Work out the finished part from the listing and answer in its coordinate system (mm). Give positions to 0.01 mm unless a question says otherwise; leave off trailing zeros. Order: outer loops, then holes, each group sorted by start corner. A loop starts at its lowest first (then second) coordinate and runs counter-clockwise, first axis right, second up. Notation, with made-up numbers: (32, 57) -> (66, 57) arc R26 cw to (66, 77) -> close; hole circle Ø11 at (51.5, 41). An arc over 180 degrees is marked (long way). Answer as CSV lines item,"result". Start each with the question number.
1. A cutting plane is placed at C-C (y = 2). State how many separate pieces and enclosed holes the cut face has, then the cut area to 3 significant figures.
2. A cutting plane is placed at D-D (z = -38). Give the vertices of the cut face in (x, y), then the cut area to 3 significant figures.
3. A cutting plane is placed at A-A (z = 27.5). Give the vertices of the cut face in (x, y).
4. A cutting plane is placed at B-B (x = -16). Give the vertices of the cut face in (y, z) (3 decimals), then the cut area to 3 significant figures.
5. Find the intervals of material crossed by L1, parallel to Z at x = -16, y = 1.9 (3 decimals); L2, parallel to Z at x = 4.5, y = 2.25; L3, parallel to Z at x = -32.5, y = 2.65, in increasing order.
6. Flat-ended cylindrical pins translate along their axes: pin 1 (2.5 mm diameter, centred on x = 30, z = 54, fed in from +Y); pin 2 (2.5 mm diameter, centred on x = -32, z = 55, fed in from +Y); pin 3 (0.9 mm diameter, centred on y = 2, z = 0.5, fed in from +X); pin 4 (1.5 mm diameter, centred on y = 1, z = -17, fed in from -X). Find the tip coordinate at first contact, or state that the pin passes through.
Autodesk Inventor part; units mm, degrees
ref_plane "YZ Plane" through (0, 0, 0) normal (1, 0, 0) x (0, 1, 0)
ref_plane "XZ Plane" through (0, 0, 0) normal (0, 1, 0) x (-1, 0, 0)
ref_plane "XY Plane" through (0, 0, 0) normal (0, 0, 1) x (1, 0, 0)
sketch "Sketch1" plane through (0, 0, 0) normal (0, 1, 0) x (-1, 0, 0)
  line L0 (32, 55) -> (-32, 55)
  line L1 (-32, 55) -> (-32, -55)
  line L2 (-32, -55) -> (32, -55)
  line L3 (32, -55) -> (32, 55)
  line L4 (32, 55) -> (-32, -55) construction
  line L5 (-32, 55) -> (32, -55) construction
  circle A0 centre (32, 55) radius 4.2425
  circle A1 centre (32, -55) radius 4.2425
  circle A2 centre (-32, 55) radius 4.2425
  circle A3 centre (-32, -55) radius 4.2425
  point P0 (0, 0)
  dimension "d0" = 64
  dimension "d1" = 110
  dimension "d2" = 8.485
  dimension "d5" = 110
  dimension "d8" = 64
extrude "Extrusion1" add sketch "Sketch1" along normal blind 3
sketch "Sketch2" plane through (0, 3, 0) normal (0, 1, 0) x (1, 0, 0)
  line L0 (32, -50.7575) -> (32, 50.7575)
  arc A0 (32, 50.7575) -> (27.7575, 55) centre (32, 55) ccw
  line L1 (27.7575, 55) -> (-27.7575, 55)
  arc A1 (-27.7575, 55) -> (-32, 50.7575) centre (-32, 55) ccw
  line L2 (-32, 50.7575) -> (-32, -50.7575)
  arc A2 (-32, -50.7575) -> (-27.7575, -55) centre (-32, -55) ccw
  line L3 (-27.7575, -55) -> (27.7575, -55)
  arc A3 (27.7575, -55) -> (32, -50.7575) centre (32, -55) ccw
  circle A4 centre (-32, -55) radius 2.15
  circle A5 centre (-32, 55) radius 2.15
  circle A6 centre (32, -55) radius 2.15
  circle A7 centre (32, 55) radius 2.15
  point P0 (0, 0)
  dimension "d13" = 4.3
  dimension "d16" = 110
  dimension "d19" = 64
extrude "Extrusion2" cut sketch "Sketch2" against normal blind 3 contours A4 | A5 | A6 | A7
sketch "Sketch3" plane through (0, 3, 0) normal (0, 1, 0) x (1, 0, 0)
  line L0 (-8, -38.5) -> (8, -38.5)
  line L1 (8, -38.5) -> (8, -5.5)
  line L2 (8, -5.5) -> (-8, -5.5)
  line L3 (-8, -5.5) -> (-8, -38.5)
  line L4 (-32, 50.7575) -> (-32, -50.7575)
  line L5 (32, -50.7575) -> (32, 50.7575)
  line L6 (-27.7575, -55) -> (27.7575, -55)
  point P0 (0, 0)
  dimension "d24" = 16
  dimension "d25" = 33
  dimension "d26" = 24
  dimension "d27" = 24
  dimension "d28" = 16.5
extrude "Extrusion3" cut sketch "Sketch3" against normal blind 3
sketch "Sketch4" plane through (0, 3, 0) normal (0, 1, 0) x (1, 0, 0)
  circle A0 centre (-16, 9.625) radius 3.4
  line L0 (0, 82.9395) -> (0, -82.9395)
  circle A1 centre (-16, 24.75) radius 3.4
  circle A2 centre (-16, 39.875) radius 3.4
  line L1 (27.7575, 55) -> (-27.7575, 55)
  line L2 (-8, -5.5) -> (8, -5.5)
  line L3 (-16, 0) -> (-16, 55)
  circle A3 centre (9, 25) radius 6
  line L4 (32, -50.7575) -> (32, 50.7575)
  point P0 (0, 0)
  dimension "d31" = 6.8
  dimension "d32" = 6.8
  dimension "d33" = 6.8
  dimension "d34" = 15.125
  dimension "d35" = 15.125
  dimension "d36" = 15.125
  dimension "d37" = 15.125
  dimension "d53" = 16
  dimension "d54" = 55
  dimension "d55" = 12
  dimension "d56" = 23
  dimension "d64" = 30
extrude "Extrusion4" cut sketch "Sketch4" against normal blind 6
sketch "Sketch5" plane through (0, 3, 0) normal (0, 1, 0) x (1, 0, 0)
  circle A0 centre (-16, 24.75) radius 3.4
  circle A1 centre (-16, 9.625) radius 3.4
  circle A2 centre (-16, 39.875) radius 3.4
  line L0 (8, -5.5) -> (8, -38.5)
  line L1 (8, -38.5) -> (-8, -38.5)
  line L2 (-8, -38.5) -> (-8, -5.5)
  line L3 (-8, -5.5) -> (8, -5.5)
  circle A3 centre (32, -55) radius 2.15
  circle A4 centre (-32, -55) radius 2.15
  circle A5 centre (-32, 55) radius 2.15
  circle A6 centre (32, 55) radius 2.15
  line L4 (32, -50.7575) -> (32, 50.7575)
  arc A7 (32, 50.7575) -> (27.7575, 55) centre (32, 55) ccw
  line L5 (27.7575, 55) -> (-27.7575, 55)
  arc A8 (-27.7575, 55) -> (-32, 50.7575) centre (-32, 55) ccw
  line L6 (-32, 50.7575) -> (-32, -50.7575)
  arc A9 (-32, -50.7575) -> (-27.7575, -55) centre (-32, -55) ccw
  line L7 (-27.7575, -55) -> (27.7575, -55)
  arc A10 (27.7575, -55) -> (32, -50.7575) centre (32, -55) ccw
  circle A11 centre (-32, -55) radius 2.15
  circle A12 centre (-32, -55) radius 4.2425
  circle A13 centre (-32, 55) radius 4.2425
  circle A14 centre (32, -55) radius 4.2425
  circle A15 centre (32, 55) radius 4.2425
  line L8 (-32, -50.7575) -> (-32, 50.7575)
  line L9 (-27.7575, 55) -> (27.7575, 55)
  line L10 (32, -50.7575) -> (32, 50.7575)
  line L11 (32, 50.7575) -> (32, -50.7575)
  line L12 (-27.7575, -55) -> (27.7575, -55)
  line L13 (27.7575, -55) -> (-27.7575, -55)
  circle A16 centre (-16, 39.875) radius 3.4
  circle A17 centre (-16, 9.625) radius 3.4
  circle A18 centre (-16, 24.75) radius 3.4
  circle A19 centre (9, 25) radius 6
  line L14 (8, -38.5) -> (8, -5.5)
  line L15 (8, -5.5) -> (-8, -5.5)
  line L16 (-8, -5.5) -> (-8, -38.5)
  line L17 (-8, -38.5) -> (8, -38.5)
  circle A20 centre (32, -55) radius 2.15
  circle A21 centre (-32, -55) radius 2.15
  circle A22 centre (-32, 55) radius 2.15
  circle A23 centre (32, 55) radius 2.15
  line L18 (-27.7575, -55) -> (27.7575, -55)
  arc A24 (-32, -50.7575) -> (-27.7575, -55) centre (-32, -55) ccw
  line L19 (-32, 50.7575) -> (-32, -50.7575)
  arc A25 (-27.7575, 55) -> (-32, 50.7575) centre (-32, 55) ccw
  line L20 (27.7575, 55) -> (-27.7575, 55)
  arc A26 (32, 50.7575) -> (27.7575, 55) centre (32, 55) ccw
  line L21 (32, -50.7575) -> (32, 50.7575)
  arc A27 (27.7575, -55) -> (32, -50.7575) centre (32, -55) ccw
  circle A28 centre (9, 25) radius 6
  point P0 (0, 0)
  dimension "d42" = 110
  dimension "d45" = 64
extrude "Extrusion6" add sketch "Sketch5" along normal blind 1.5 contours A14 L7 A12 L6 A13 L5 A15 L4
chamfer "Chamfer2" distance 1.5 angle 45 4 edges at (-32, 4.5, 0) (0, 4.5, 55) (32, 4.5, 0) (0, 4.5, -55)
equation "\"d26\" = d27"
equation "\"d32\" = d31"
equation "\"d33\" = d31"
equation "\"d34\" = d37"
equation "\"d35\" = d34"
equation "\"d36\" = d34"
properties part number "gora"
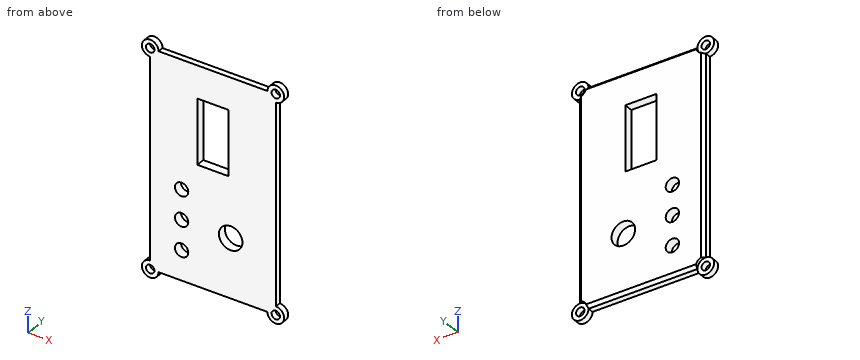
Answer sheet:
1,separate pieces,"1"
1,enclosed holes,"9"
1,area,"6,400 mm^2"
2,outline,"(-32, 0) -> (-18.84, 0) -> (-18.84, 4.5) -> (-30.5, 4.5) -> (-32, 3) -> close; (-13.16, 0) -> (32, 0) -> (32, 3) -> (30.5, 4.5) -> (-13.16, 4.5) -> close"
2,area,"260 mm^2"
3,outline,"(-32, 0) -> (-8, 0) -> (-8, 4.5) -> (-30.5, 4.5) -> (-32, 3) -> close; (8, 0) -> (32, 0) -> (32, 3) -> (30.5, 4.5) -> (8, 4.5) -> close"
4,outline,"(0, -55) -> (3, -55) -> (4.5, -53.5) -> (4.5, -43.275) -> (0, -43.275) -> close; (0, -36.475) -> (4.5, -36.475) -> (4.5, -28.15) -> (0, -28.15) -> close; (0, -21.35) -> (4.5, -21.35) -> (4.5, -13.025) -> (0, -13.025) -> close; (0, -6.225) -> (4.5, -6.225) -> (4.5, 53.5) -> (3, 55) -> (0, 55) -> close"
4,area,"401 mm^2"
5,L1,"z = -55 to -43.275, -36.475 to -28.15, -21.35 to -13.025, -6.225 to 55"
5,L2,"z = -55 to -28.97, -21.03 to 5.5, 38.5 to 55"
5,L3,"z = -59.21 to -57.09, -52.91 to -50.79, 50.79 to 52.91, 57.09 to 59.21"
6,pin 1,"stops at y = 3"
6,pin 2,"passes through"
6,pin 3,"stops at x = 32"
6,pin 4,"stops at x = -32"
